```python
from build123d import *

# Parameters (mm, degrees)
F0_W      = 65
F0_H      = 45
F1_DEPTH  = 5
F2_W      = 65
F2_H      = 45
F2_W_2    = 60
F2_H_2    = 40
F3_DEPTH  = 10
F4_W      = 19.5
F4_H      = 1
F4_W_2    = 1
F4_H_2    = 19.5
F4_W_3    = 19
F5_DEPTH  = 1
F7_DEPTH  = 1
F11_DEPTH = 1
F9_W      = 1
F9_H      = 11
F12_DEPTH = 1
F8_W      = 1
F8_H      = 11
F13_DEPTH = 1
F14_W     = 10
F14_H     = 10
F15_DEPTH = 9


with BuildPart() as f1:
    # F0 (on Top) → F1 (new body)
    with BuildSketch(Plane.XY):
        Rectangle(F0_W, F0_H)
    extrude(amount=F1_DEPTH)

    # F2 (on face) → F3 (join)
    with BuildSketch(Plane.XY.offset(5)):
        Rectangle(F2_W, F2_H)
        Rectangle(F2_W_2, F2_H_2, mode=Mode.SUBTRACT)
    extrude(amount=F3_DEPTH)

    # F4 (on face) → F5 (cut)
    with BuildSketch(Plane.XY.offset(5)):
        with Locations((-20.25, 0)):
            Rectangle(F4_W, F4_H)
        with Locations((-10, 0)):
            Rectangle(F4_W_2, F4_H)
        with Locations((-10, 10.25)):
            Rectangle(F4_W_2, F4_H_2)
        with Locations((-10, -10.25)):
            Rectangle(F4_W_2, F4_H_2)
        Rectangle(F4_W_3, F4_H)
        with Locations((10, 10.25)):
            Rectangle(F4_W_2, F4_H_2)
        with Locations((10, -10.25)):
            Rectangle(F4_W_2, F4_H_2)
        with Locations((20.25, 0)):
            Rectangle(F4_W, F4_H)
        with Locations((10, 0)):
            Rectangle(F4_W_2, F4_H)
    extrude(amount=-F5_DEPTH, mode=Mode.SUBTRACT)

    # F6 (on face) → F7 (cut)
    with BuildSketch(Plane.XZ.offset(-20)):
        Polygon((-10.5, 5), (-10.5, 4), (-9.5, 4), (-9.5, 5), (-9.5, 15), (-10.5, 15), align=None)
        Polygon((9.5, 15), (9.5, 5), (9.5, 4), (10.5, 4), (10.5, 5), (10.5, 15), align=None)
    extrude(amount=-F7_DEPTH, mode=Mode.SUBTRACT)

    # F10 (on face) → F11 (cut)
    with BuildSketch(Plane.YZ.offset(-30)):
        Polygon((-0.5, 5), (-0.5, 4), (0.5, 4), (0.5, 5), (0.5, 15), (-0.5, 15), align=None)
    extrude(amount=-F11_DEPTH, mode=Mode.SUBTRACT)

    # F9 (on face) → F12 (cut)
    with BuildSketch(Plane(origin=(0, -20, 0), x_dir=(-1, 0, 0), z_dir=(0, 1, 0))):
        with Locations((-10, 9.5)):
            Rectangle(F9_W, F9_H)
        with Locations((10, 9.5)):
            Rectangle(F9_W, F9_H)
    extrude(amount=-F12_DEPTH, mode=Mode.SUBTRACT)

    # F8 (on face) → F13 (cut)
    with BuildSketch(Plane(origin=(30, 0, 0), x_dir=(0, -1, 0), z_dir=(-1, 0, 0))):
        with Locations((0, 9.5)):
            Rectangle(F8_W, F8_H)
    extrude(amount=-F13_DEPTH, mode=Mode.SUBTRACT)

    # F14 (on face) → F15 (join)
    with BuildSketch(Plane.XY.offset(5)):
        with Locations((-20, 10)):
            Rectangle(F14_W, F14_H)
        with Locations((0, 10)):
            Rectangle(F14_W, F14_H)
        with Locations((20, 10)):
            Rectangle(F14_W, F14_H)
        with Locations((20, -10)):
            Rectangle(F14_W, F14_H)
        with Locations((0, -10)):
            Rectangle(F14_W, F14_H)
        with Locations((-20, -10)):
            Rectangle(F14_W, F14_H)
    extrude(amount=F15_DEPTH)


solid = f1.part
```
Here's how the part is built. I have some questions about the finished solid (model axes, mm). A direction names the side the tool comes from. Coordinates: 2 decimals unless noted, no trailing zeros. Order: outer loops, then holes, each group sorted by start corner. A loop starts at its lowest first (then second) coordinate and runs counter-clockwise, first axis right, second up. Notation, with made-up numbers: (11.5, -39) - (21.5, -39) arc R31 cw to (21.5, -12) - close; hole circle Ø6 at (79, 67). An arc over 180 degrees is marked (long way). One line per question, with ' | ' between items. Start each with the question number.
1. If we section it at A-A (z = 12.5): Give the number of separate pieces and of enclosed holes in the cut face, and give its area (3 significant figures).
2. I'm going to push flat-ended pins straight in: pin 1 Ø15.5 at (x, y) = (-19.5, -6) entering from +Z; pin 2 Ø2 at (x, y) = (-16.5, -18) entering from +Z. Where does each tip first touch, or does it pass through?
3. Which directions (+Z, -Z, +X, -X, +Y, -Y) give clear straight access to the entire face, cutting with the end or side of a thin tool? Please do faces 1 (the flat face through (0, 0, 0)), 2 (the flat face through (-5, 10, 9)).
4. Please list where these lines run through material, in increasing order: line 1 along X through (y, z) = (12, 6.5); line 2 along Y through (x, z) = (17, 7.75); line 3 along Y through (x, z) = (19, 14.25). Write a range as [from, to].
5. If we section it at B-B (x = -3.5): Write out the boundary of the cut face in (y, z), and give its area (3 significant figures).
6. If we mould it in two halves opening along X, with no side actions, what happens to faces 3 (the flat face through (0, 10, 14)), 4 (the flat face through (0, -22.5, 7))? For each: released by +X, released by -X, zero draft, split by the parting line, or undercut.
7. If we section it at D-D (x = 12): Write out the boundary of the cut face in (y, z), and give its area (3 significant figures).
8. If we section it at C-C (y = 10): Write out the boundary of the cut face in (x, z).
Model answer:
1) separate pieces: 7 | enclosed holes: 1 | area: 1,120 mm²
2) pin 1: stops at z = 14 | pin 2: stops at z = 5
3) face 1: -Z, +X, -X, +Y, -Y | face 2: +Z
4) line 1: x = [-32.5, -30], [-25, -15], [-5, 5], [15, 25], [30, 32.5] | line 2: y = [-22.5, -20], [-15, -5], [5, 15], [20, 22.5] | line 3: y = [-22.5, -20], [20, 22.5]
5) outline: (-22.5, 0) - (22.5, 0) - (22.5, 15) - (20, 15) - (20, 5) - (15, 5) - (15, 14) - (5, 14) - (5, 5) - (0.5, 5) - (0.5, 4) - (-0.5, 4) - (-0.5, 5) - (-5, 5) - (-5, 14) - (-15, 14) - (-15, 5) - (-20, 5) - (-20, 15) - (-22.5, 15) - close | area: 454 mm²
6) face 3: undercut | face 4: zero draft
7) outline: (-22.5, 0) - (22.5, 0) - (22.5, 15) - (20, 15) - (20, 5) - (0.5, 5) - (0.5, 4) - (-0.5, 4) - (-0.5, 5) - (-20, 5) - (-20, 15) - (-22.5, 15) - close | area: 274 mm²
8) outline: (-32.5, 0) - (32.5, 0) - (32.5, 15) - (30, 15) - (30, 5) - (25, 5) - (25, 14) - (15, 14) - (15, 5) - (10.5, 5) - (10.5, 4) - (9.5, 4) - (9.5, 5) - (5, 5) - (5, 14) - (-5, 14) - (-5, 5) - (-9.5, 5) - (-9.5, 4) - (-10.5, 4) - (-10.5, 5) - (-15, 5) - (-15, 14) - (-25, 14) - (-25, 5) - (-30, 5) - (-30, 15) - (-32.5, 15) - close
